Work out the finished part from the listing and answer in its coordinate system (mm). A direction names the side the tool comes from. Coordinates: 2 decimals unless noted, no trailing zeros. Order: outer loops, then holes, each group sorted by start corner. A loop starts at its lowest first (then second) coordinate and runs counter-clockwise, first axis right, second up. Notation, with made-up numbers: M -24.75,-29.5 L -14.75,-29.5 A15 ccw -14.75,-15.5 Z; hole C 35.5,11.25 d10. An arc over 180 degrees is marked long. Use a Markdown table: item, result.
from build123d import *

# Parameters (mm, degrees)
BOSS_EXTRUDE1_DEPTH                             = 12.7
M4X0_7_TAPPED_HOLE1_D                           = 3.3
M8X1_25_TAPPED_HOLE1_D                          = 6.8
CSK_FOR_M6_FLAT_HEAD_MACHINE_SCREW1_D           = 6.4
CSK_FOR_M6_FLAT_HEAD_MACHINE_SCREW1_CSINK_D     = 12.6
CSK_FOR_M6_FLAT_HEAD_MACHINE_SCREW1_CSINK_ANGLE = 90
M6X1_0_TAPPED_HOLE2_D                           = 5
M6X1_0_TAPPED_HOLE2_DEPTH                       = 15
M6X1_0_TAPPED_HOLE2_TIP                         = 1.502151548
M6X1_0_TAPPED_HOLE1_D                           = 5
M6X1_0_TAPPED_HOLE1_DEPTH                       = 15
M6X1_0_TAPPED_HOLE1_TIP                         = 1.502151548
CSK_FOR_M6_FLAT_HEAD_MACHINE_SCREW2_D           = 6.4
CSK_FOR_M6_FLAT_HEAD_MACHINE_SCREW2_CSINK_D     = 12.6
CSK_FOR_M6_FLAT_HEAD_MACHINE_SCREW2_CSINK_ANGLE = 90
F_1_3_4_CLEARANCE_HOLE1_D                       = 45
F_1_3_4_CLEARANCE_HOLE1_DEPTH                   = 5
M6_CLEARANCE_HOLE1_D                            = 6.6
FILLET1_R                                       = 44.45


with BuildPart() as part:
    # Sketch1 → Boss-Extrude1 (new body)
    with BuildSketch(Plane(origin=(0, 0, 0), x_dir=(-1, 0, 0), z_dir=(0, 0, -1))):
        with BuildLine():
            Line((-6, -44.45), (44.45, -44.45))
            Line((44.45, -44.45), (44.45, 60))
            Line((44.45, 60), (-44.45, 60))
            Line((-44.45, 60), (-44.45, 0))
            Line((-44.45, 0), (-50.45, 0))
            ThreePointArc((-50.45, 0), (-37.430896424, -31.430896424), (-6, -44.45))
        make_face()
    extrude(amount=-BOSS_EXTRUDE1_DEPTH)

    # M4x0.7 Tapped Hole1 (through all)
    with Locations(Plane.XY.offset(12.7)):
        with Locations((32.349998458, 0.009014041), (6, -26.35), (-20.349998115, -0.009967087), (6, 26.35)):
            Hole(M4X0_7_TAPPED_HOLE1_D / 2)

    # M8x1.25 Tapped Hole1 (through all)
    with Locations(Plane.XY.offset(12.7)):
        with Locations((17.47250377, 49.692873304)):
            Hole(M8X1_25_TAPPED_HOLE1_D / 2)

    # CSK for M6 Flat Head Machine Screw1 (through all)
    with Locations(Plane(origin=(0, 0, 0), x_dir=(-1, 0, 0), z_dir=(0, 0, -1))):
        with Locations((23.65, 22)):
            CounterSinkHole(CSK_FOR_M6_FLAT_HEAD_MACHINE_SCREW1_D / 2, CSK_FOR_M6_FLAT_HEAD_MACHINE_SCREW1_CSINK_D / 2, counter_sink_angle=CSK_FOR_M6_FLAT_HEAD_MACHINE_SCREW1_CSINK_ANGLE)

    # M6x1.0 Tapped Hole2
    with Locations(Plane(origin=(44.45, 0, 0), x_dir=(0, 0, -1), z_dir=(1, 0, 0))):
        with Locations((-6.35, 7), (-6.35, 53), (-6.35, 30)):
            Hole(M6X1_0_TAPPED_HOLE2_D / 2, depth=M6X1_0_TAPPED_HOLE2_DEPTH)
            with Locations((0, 0, -(M6X1_0_TAPPED_HOLE2_DEPTH + M6X1_0_TAPPED_HOLE2_TIP / 2))):  # 118° drill point
                Cone(0, M6X1_0_TAPPED_HOLE2_D / 2, M6X1_0_TAPPED_HOLE2_TIP, mode=Mode.SUBTRACT)

    # M6x1.0 Tapped Hole1
    with Locations(Plane(origin=(0, 60, 0), x_dir=(1, 0, 0), z_dir=(0, 1, 0))):
        with Locations((-38.45, -6.35), (-8.85, -6.35)):
            Hole(M6X1_0_TAPPED_HOLE1_D / 2, depth=M6X1_0_TAPPED_HOLE1_DEPTH)
            with Locations((0, 0, -(M6X1_0_TAPPED_HOLE1_DEPTH + M6X1_0_TAPPED_HOLE1_TIP / 2))):  # 118° drill point
                Cone(0, M6X1_0_TAPPED_HOLE1_D / 2, M6X1_0_TAPPED_HOLE1_TIP, mode=Mode.SUBTRACT)

    # CSK for M6 Flat Head Machine Screw2 (through all)
    with Locations(Plane(origin=(0, 0, 0), x_dir=(-1, 0, 0), z_dir=(0, 0, -1))):
        with Locations((38.45, 30), (38.45, 6)):
            CounterSinkHole(CSK_FOR_M6_FLAT_HEAD_MACHINE_SCREW2_D / 2, CSK_FOR_M6_FLAT_HEAD_MACHINE_SCREW2_CSINK_D / 2, counter_sink_angle=CSK_FOR_M6_FLAT_HEAD_MACHINE_SCREW2_CSINK_ANGLE)

    # 1-3/4 Clearance Hole1
    with Locations(Plane(origin=(0, 0, 0), x_dir=(-1, 0, 0), z_dir=(0, 0, -1))):
        with Locations((-6, 0)):
            Hole(F_1_3_4_CLEARANCE_HOLE1_D / 2, depth=F_1_3_4_CLEARANCE_HOLE1_DEPTH)

    # M6 Clearance Hole1 (through all)
    with Locations(Plane.XY.offset(12.7)):
        with Locations((6, 17.5), (22.643489035, 5.407797402), (16.286241915, -14.157797402), (-4.286241915, -14.157797402), (-10.643489035, 5.407797402)):
            Hole(M6_CLEARANCE_HOLE1_D / 2)

    # Fillet1
    fillet1_edges = [part.edges().sort_by_distance(p)[0] for p in [
        (-44.45, -44.45, 6.35),
    ]]
    fillet(fillet1_edges, radius=FILLET1_R)


solid = part.part
(1) Given P1, Ø5.5, axis at x = 6, y = 17.5, coming from the +Z side; P2, Ø6, axis at y = -3.5, z = 8, coming from the -X side; P3, Ø4, axis at y = 6.5, z = 2.5, coming from the +X side; P4, Ø7.5, axis at x = 16.29, y = -14.16, coming from the -Z side, each flat-ended and moving along its own axis, determine where each tip first touches the part or whether it passes through.
Conclusion:
| item | result |
|---|---|
| P1 | through |
| P2 | x = -44.45 |
| P3 | x = 44.45 |
| P4 | z = 5 |
(2) A cutting plane is placed at B-B (z = 10.5). Give the number of separate pieces and of enclosed holes in the cut face, then the cut area to 3 significant figures.
Conclusion:
| item | result |
|---|---|
| separate pieces | 1 |
| enclosed holes | 13 |
| area | 8,370 mm2 |
(3) Which of the six approach directions +Z, -Z, +X, -X, +Y, -Y give full straight-line access (tool end or side, diameter ignored) to faces 1 (the cylindrical face through (-6.352, 52.395, 6.24)), 2 (the flat face through (-1, 60, 6)), 3 (the cylindrical face through (-35.398, 6.961, 7.967)), 4 (the flat face through (6, 0, 5)), 5 (the flat face through (47, 0, 6))?
Conclusion:
| item | result |
|---|---|
| face 1 | +Y |
| face 2 | +Z, -Z, +X, -X, +Y |
| face 3 | +Z, -Z |
| face 4 | -Z |
| face 5 | +Z, -Z, +X, +Y |
(4) Determine the mould class of faces 6 (the cylindrical face through (30.776, 0.505, 6.261)), 7 (the conical face through (28.21, 7.37, 6.12)), 8 (the cylindrical face through (36.84, 31.69, 4.51)) for opening direction X: pulls with the +X half, pulls with the -X half, needs draft (parallel to the pull), parting line crosses it, or undercut.
Conclusion:
| item | result |
|---|---|
| face 6 | undercut |
| face 7 | pulls with the +X half |
| face 8 | needs draft |
(5) Straight lines are drawn through the part: L1, parallel to Y at x = 6, z = 4.75; L2, parallel to X at y = 3.5, z = 2; L3, parallel to Y at x = 40, z = 7. For each, find the intervals that lie inside material, in ascending order.
Conclusion:
| item | result |
|---|---|
| L1 | -44.45 to -28, -24.7 to -22.5, 22.5 to 24.7, 28 to 60 |
| L2 | -44.45 to -41.95, -34.95 to -16.23, 28.23 to 44.45 |
| L3 | -28.63 to 4.59, 9.41 to 27.59, 32.41 to 50.59, 55.41 to 60 |
(6) A cutting plane is placed at A-A (x = -23.65). Determine the outline of the cut face in (y, z).
Conclusion:
| item | result |
|---|---|
| outline | M -37.64,0 L 15.7,0 L 18.8,3.1 L 18.8,12.7 L -37.64,12.7 Z; M 25.2,3.1 L 28.3,0 L 60,0 L 60,12.7 L 25.2,12.7 Z |
(7) A cutting plane is placed at C-C (y = -36). Determine the outline of the cut face in (x, z), then the cut area to 3 significant figures.
Conclusion:
| item | result |
|---|---|
| outline | M -26.07,0 L 32.07,0 L 32.07,12.7 L -26.07,12.7 Z |
| area | 738 mm2 |
